from build123d import *

# Parameters (mm, degrees)
SKETCH_1_W               = 57
SKETCH_1_H               = 57
SKETCH_1_R               = 2.5
EXTRUDE_1_DEPTH          = 90
CUT_EXTRUDE_1_DEPTH      = 35
CUT_EXTRUDE_1_DEPTH_BACK = 25
SKETCH_2_W               = 108.428047284
SKETCH_2_H               = 112.732753546
SKETCH_2_R               = 28.5
SKETCH_3_R               = 21
EXTRUDE_2_DEPTH          = 3
SKETCH_4_R               = 7
EXTRUDE_3_DEPTH          = 20
SKETCH_5_R               = 4
CUT_EXTRUDE_2_DEPTH      = 26
SKETCH_6_R               = 19.05
CUT_EXTRUDE_3_DEPTH      = 3
EXTRUDE_4_DEPTH          = 18


with BuildPart() as part:
    # 草图1 → 凸台-拉伸1 (new body)
    with BuildSketch(Plane.XY):
        Rectangle(SKETCH_1_W, SKETCH_1_H)
        with Locations(Location((-23.57, 23.57, 0), (0, 0, 180))):
            Circle(SKETCH_1_R, mode=Mode.SUBTRACT)
        with Locations(Location((23.57, 23.57, 0), (0, 0, 180))):
            Circle(SKETCH_1_R, mode=Mode.SUBTRACT)
        with Locations(Location((23.57, -23.57, 0), (0, 0, 180))):
            Circle(SKETCH_1_R, mode=Mode.SUBTRACT)
        with Locations(Location((-23.57, -23.57, 0), (0, 0, 180))):
            Circle(SKETCH_1_R, mode=Mode.SUBTRACT)
    extrude(amount=EXTRUDE_1_DEPTH)

    # 草图2 → 切除-拉伸1 (cut, two sides: drawn at the far end of the back side and taken through both)
    with BuildSketch(Plane(origin=(0, 0, 45), x_dir=(-1, 0, 0), z_dir=(0, 0, -1)).offset(-CUT_EXTRUDE_1_DEPTH_BACK)):
        Rectangle(SKETCH_2_W, SKETCH_2_H)
        with Locations(Location((0, 0, 0), (0, 0, 180))):
            Circle(SKETCH_2_R, mode=Mode.SUBTRACT)
    extrude(amount=CUT_EXTRUDE_1_DEPTH + CUT_EXTRUDE_1_DEPTH_BACK, mode=Mode.SUBTRACT)

    # 草图3 → 凸台-拉伸2 (add)
    with BuildSketch(Plane(origin=(0, 0, 0), x_dir=(-1, 0, 0), z_dir=(0, 0, -1))):
        Circle(SKETCH_3_R)
    extrude(amount=EXTRUDE_2_DEPTH)

    # 草图4 → 凸台-拉伸3 (add)
    with BuildSketch(Plane(origin=(0, 0, -3), x_dir=(-1, 0, 0), z_dir=(0, 0, -1))):
        Circle(SKETCH_4_R)
    extrude(amount=EXTRUDE_3_DEPTH)

    # 草图5 → 切除-拉伸2 (cut)
    with BuildSketch(Plane.XY.offset(90)):
        Circle(SKETCH_5_R)
    extrude(amount=-CUT_EXTRUDE_2_DEPTH, mode=Mode.SUBTRACT)

    # 草图6 → 切除-拉伸3 (cut)
    with BuildSketch(Plane.XY.offset(90)):
        Circle(SKETCH_6_R)
    extrude(amount=-CUT_EXTRUDE_3_DEPTH, mode=Mode.SUBTRACT)

    # 草图7 → 凸台-拉伸4 (add)
    with BuildSketch(Plane(origin=(0, 0, -23), x_dir=(-1, 0, 0), z_dir=(0, 0, -1))):
        Polygon((0, 9), (2.5, 9), (2.5, 0), (-2.5, 0), (-2.5, 9), align=None)
    extrude(amount=-EXTRUDE_4_DEPTH)


solid = part.part
Verification items for the finished model (mm, model axes). A direction names the side the tool comes from. Coordinates: 2 decimals unless noted, no trailing zeros. Order: outer loops, then holes, each group sorted by start corner. A loop starts at its lowest first (then second) coordinate and runs counter-clockwise, first axis right, second up.
1. Go/stop test with flat-tipped pins: pin 1 Ø3 at (x, y) = (-23.57, -23.57) entering from +Z; pin 2 Ø10 at (y, z) = (-6.5, 37.5) entering from -X; pin 3 Ø9 at (x, y) = (-1, 1) entering from +Z; pin 4 Ø10 at (x, z) = (-8, 40.5) entering from +Y. Record where each tip stops, or that it passes through.
Results found:
pin 1: passes through
pin 2: stops at x = -28.46
pin 3: stops at z = 87
pin 4: stops at y = 28.34
2. Scan lines: line 1 (Y direction, x = 23.57, z = 74); line 2 (Z direction, x = -13, y = 3.5). Record each from-to range of solid material in increasing order.
Results found:
line 1: y = -28.5 to -26.07, -21.07 to 21.07, 26.07 to 28.5
line 2: z = -3 to 87
3. Release check for a two-part mould opening along Y. For faces 5 (the face through (-21.586, 25.091, 4.93)), 6 (the face through (28.5, 0, 80)), 7 (the face through (0, 28.5, 80)) record: +Y half, -Y half, draft (parallel to the pull), parting line (faces both ways), or undercut.
Results found:
face 5: undercut
face 6: draft
face 7: +Y half
4. Set-up check for faces 1 (the face through (0, 0, 64)), 2 (the face through (21.7, -21.6, 70)), 3 (the face through (-20.03, 6.31, -1.48)), 4 (the face through (-21, -22, 10)): record each of +Z, -Z, +X, -X, +Y, -Y from which the full face is reachable in a straight line by a thin tool's end or side.
Results found:
face 1: +Z
face 2: +X, -Y
face 3: -Z
face 4: -X, -Y
5. Sectioned sample at B-B, the plane x = -23.57. Record the cut outline in (y, z), and give its area (3 significant figures).
Results found:
outline: (-28.5, 0) - (-26.07, 0) - (-26.07, 10) - (-28.5, 10) - close; (-28.5, 70) - (-26.07, 70) - (-26.07, 90) - (-28.5, 90) - close; (-21.07, 0) - (21.07, 0) - (21.07, 10) - (16.02, 10) - (16.02, 70) - (21.07, 70) - (21.07, 90) - (-21.07, 90) - (-21.07, 70) - (-16.02, 70) - (-16.02, 10) - (-21.07, 10) - close; (26.07, 0) - (28.5, 0) - (28.5, 10) - (26.07, 10) - close; (26.07, 70) - (28.5, 70) - (28.5, 90) - (26.07, 90) - close
area: 3,330 mm2
6. Sectioned sample at D-D, the plane y = 11.5. Record the cut outline in (x, z).
Results found:
outline: (-28.5, 0) - (-17.57, 0) - (-17.57, -3) - (17.57, -3) - (17.57, 0) - (28.5, 0) - (28.5, 10) - (26.08, 10) - (26.08, 70) - (28.5, 70) - (28.5, 90) - (15.19, 90) - (15.19, 87) - (-15.19, 87) - (-15.19, 90) - (-28.5, 90) - (-28.5, 70) - (-26.08, 70) - (-26.08, 10) - (-28.5, 10) - close
7. Sectioned sample at A-A, the plane z = 72. Record the cut outline in (x, y).
Results found:
outline: (-28.5, -28.5) - (28.5, -28.5) - (28.5, 28.5) - (-28.5, 28.5) - close; hole circle Ø5 at (-23.57, -23.57); hole circle Ø5 at (-23.57, 23.57); hole circle Ø8 at (0, 0); hole circle Ø5 at (23.57, -23.57); hole circle Ø5 at (23.57, 23.57)
